Check sheet for the modelled part. Datum: model origin and axes. Units: mm. A direction names the side the tool comes from. Coordinates: 2 decimals unless noted, no trailing zeros. Order: outer loops, then holes, each group sorted by start corner. A loop starts at its lowest first (then second) coordinate and runs counter-clockwise, first axis right, second up. Notation, with made-up numbers: (-40, -39.75) -> (9, -39.75) arc R20 ccw to (9, -4.75) -> close; hole circle Ø2 at (-20, 80). An arc over 180 degrees is marked (long way). Put each result on its own line as item: value. Start each with the question number.
```python
from build123d import *

# Parameters (mm, degrees)
EXTRUDE_1_OUTLINE_R   = 150
EXTRUDE_1_OUTLINE_R_2 = 3
EXTRUDE_1_OUTLINE_R_3 = 2
EXTRUDE_1_OUTLINE_W   = 22.346122356
EXTRUDE_1_OUTLINE_H   = 26.623931282
EXTRUDE_1_DEPTH       = 3
FILLET_1_R            = 10
FILLET_2_R            = 10
FILLET_3_R            = 10
FILLET_4_R            = 10
FILLET_5_R            = 10
FILLET_6_R            = 10
FILLET_7_R            = 10
FILLET_8_R            = 10


# Read off the part's stored shape, not the designer's step: Бобышка-Вытянуть1
with BuildPart() as part:
    # Бобышка-Вытянуть1 outline → Бобышка-Вытянуть1 (new body)
    with BuildSketch(Plane(origin=(0, 0, 0), x_dir=(1, 0, 0), z_dir=(0, 1, 0))):
        Circle(EXTRUDE_1_OUTLINE_R)
        with Locations((-102.530483272, -102.530483272)):
            Circle(EXTRUDE_1_OUTLINE_R_2, mode=Mode.SUBTRACT)
        with Locations((-10, -10)):
            Circle(EXTRUDE_1_OUTLINE_R_3, mode=Mode.SUBTRACT)
        with Locations((0, -145)):
            Circle(EXTRUDE_1_OUTLINE_R_2, mode=Mode.SUBTRACT)
        with Locations((102.530483272, -102.530483272)):
            Circle(EXTRUDE_1_OUTLINE_R_2, mode=Mode.SUBTRACT)
        with Locations((10, -10)):
            Circle(EXTRUDE_1_OUTLINE_R_3, mode=Mode.SUBTRACT)
        with Locations((-145, 0)):
            Circle(EXTRUDE_1_OUTLINE_R_2, mode=Mode.SUBTRACT)
        with Locations((-51.559180368, 0)):
            Rectangle(EXTRUDE_1_OUTLINE_W, EXTRUDE_1_OUTLINE_H, mode=Mode.SUBTRACT)
        with Locations((-10, 10)):
            Circle(EXTRUDE_1_OUTLINE_R_3, mode=Mode.SUBTRACT)
        with Locations((-102.530483272, 102.530483272)):
            Circle(EXTRUDE_1_OUTLINE_R_2, mode=Mode.SUBTRACT)
        with Locations((10, 10)):
            Circle(EXTRUDE_1_OUTLINE_R_3, mode=Mode.SUBTRACT)
        with Locations((51.559180368, 0)):
            Rectangle(EXTRUDE_1_OUTLINE_W, EXTRUDE_1_OUTLINE_H, mode=Mode.SUBTRACT)
        with Locations((145, 0)):
            Circle(EXTRUDE_1_OUTLINE_R_2, mode=Mode.SUBTRACT)
        with Locations((0, 145)):
            Circle(EXTRUDE_1_OUTLINE_R_2, mode=Mode.SUBTRACT)
        with Locations((102.530483272, 102.530483272)):
            Circle(EXTRUDE_1_OUTLINE_R_2, mode=Mode.SUBTRACT)
    extrude(amount=EXTRUDE_1_DEPTH)

    # Скругление1
    fillet_1_edges = [part.edges().sort_by_distance(p)[0] for p in [
        (-62.732241546, 1.5, -13.311965641),
    ]]
    fillet(fillet_1_edges, radius=FILLET_1_R)

    # Скругление2
    fillet_2_edges = [part.edges().sort_by_distance(p)[0] for p in [
        (-40.38611919, 1.5, 13.311965641),
    ]]
    fillet(fillet_2_edges, radius=FILLET_2_R)

    # Скругление3
    fillet_3_edges = [part.edges().sort_by_distance(p)[0] for p in [
        (40.38611919, 1.5, 13.311965641),
    ]]
    fillet(fillet_3_edges, radius=FILLET_3_R)

    # Скругление4
    fillet_4_edges = [part.edges().sort_by_distance(p)[0] for p in [
        (62.732241546, 1.5, -13.311965641),
    ]]
    fillet(fillet_4_edges, radius=FILLET_4_R)

    # Скругление5
    fillet_5_edges = [part.edges().sort_by_distance(p)[0] for p in [
        (-40.38611919, 1.5, -13.311965641),
    ]]
    fillet(fillet_5_edges, radius=FILLET_5_R)

    # Скругление6
    fillet_6_edges = [part.edges().sort_by_distance(p)[0] for p in [
        (-62.732241546, 1.5, 13.311965641),
    ]]
    fillet(fillet_6_edges, radius=FILLET_6_R)

    # Скругление7
    fillet_7_edges = [part.edges().sort_by_distance(p)[0] for p in [
        (62.732241546, 1.5, 13.311965641),
    ]]
    fillet(fillet_7_edges, radius=FILLET_7_R)

    # Скругление8
    fillet_8_edges = [part.edges().sort_by_distance(p)[0] for p in [
        (40.38611919, 1.5, -13.311965641),
    ]]
    fillet(fillet_8_edges, radius=FILLET_8_R)


solid = part.part
```
1) Mould release check, pull along Z, two halves, no side actions. Record for faces 1 (the cylindrical face through (-19.527, 1.479, -148.724)), 2 (the flat face through (-2, 3, -2)), 3 (the cylindrical face through (-59.725, 1.521, 10.46)), 4 (the cylindrical face through (59.881, 1.521, -10.305)): +Z half, -Z half, draft (parallel to the pull), parting line (faces both ways), or undercut.
2) Sectioned sample at A-A (y = 0.5). State how many separate pieces and enclosed holes the cut face has, plus the area to 3 significant figures.
3) Access from +Z, -Z, +X, -X, +Y, -Y to the whole of each face (thin tool, end or side, straight path). Record for faces 5 (the cylindrical face through (43.393, 1.521, -10.46)), 6 (the flat face through (-2, 0, -2)).
4) Sectioned sample at B-B (x = 74.5). Record the boundary of the cut face in (y, z).
5) Scan lines: line 1 along X through (y, z) = (1.5, 0); line 2 along Z through (x, y) = (0, 1.4); line 3 along X through (y, z) = (0.3, 102). Record each from-to range of solid material in increasing order. Write a range as [from, to].
6) Gauge pin test, flat ends, axial feed: pin 1 (3.5 mm diameter, centred on x = -10, z = -10, fed in from +Y); pin 2 (0.7 mm diameter, centred on x = 51.5, y = 2, fed in from -Z); pin 3 (1 mm diameter, centred on x = -56.5, y = 0.5, fed in from -Z). Record the tip position at first contact, or that the pin passes through.
7) Sectioned sample at C-C (z = -81). Record the boundary of the cut face in (x, y).
Entries:
1. face 1: parting line
1. face 2: draft
1. face 3: undercut
1. face 4: undercut
2. separate pieces: 1
2. enclosed holes: 14
2. area: 69,400 mm2
3. face 5: +Y, -Y
3. face 6: +Z, -Z, +X, -X, -Y
4. outline: (0, -130.19) -> (3, -130.19) -> (3, 130.19) -> (0, 130.19) -> close
5. line 1: x = [-150, -148], [-142, -62.73], [-40.39, 40.39], [62.73, 142], [148, 150]
5. line 2: z = [-150, -148], [-142, 142], [148, 150]
5. line 3: x = [-109.98, -105.48], [-99.58, 99.58], [105.48, 109.98]
6. pin 1: passes through
6. pin 2: stops at z = -141.01
6. pin 3: stops at z = -139.15
7. outline: (-126.25, 0) -> (126.25, 0) -> (126.25, 3) -> (-126.25, 3) -> close
